Build history of the part. All positions in model axes, mm. Face numbers are marked on the shaded views. A direction names the side the tool comes from. Give positions to 0.01 mm unless a question says otherwise; leave off trailing zeros. Order: outer loops, then holes, each group sorted by start corner. A loop starts at its lowest first (then second) coordinate and runs counter-clockwise, first axis right, second up. Notation, with made-up numbers: M 0.5,22 L 59.5,22 A37 cw 59.5,60 Z; hole C -13.5,76 d6. An arc over 180 degrees is marked long. One line per item, written item: value.
from build123d import *

# Parameters (mm, degrees)
SKETCH1_W           = 96.52
SKETCH1_H           = 63.5
SKETCH1_R           = 1.905
BOSS_EXTRUDE1_DEPTH = 29.21
SKETCH2_W           = 86.36
SKETCH2_H           = 50.8
SKETCH2_W_2         = 5.705747077
SKETCH2_H_2         = 14.834942399
BOSS_EXTRUDE2_DEPTH = 2.54
SKETCH3_R           = 1.27
CUT_EXTRUDE1_DEPTH  = 2.54
SKETCH4_W           = 7.62
SKETCH4_H           = 6.35
SKETCH4_W_2         = 10.16
BOSS_EXTRUDE3_DEPTH = 10.16


with BuildPart() as part:
    # Sketch1 → Boss-Extrude1 (new body)
    with BuildSketch(Plane(origin=(0, 0, 0), x_dir=(1, 0, 0), z_dir=(0, 1, 0))):
        Rectangle(SKETCH1_W, SKETCH1_H)
        with Locations(Location((-43.18, 26.67, 0), (0, 0, 90))):
            Circle(SKETCH1_R, mode=Mode.SUBTRACT)
        with Locations(Location((43.18, 26.67, 0), (0, 0, 90))):
            Circle(SKETCH1_R, mode=Mode.SUBTRACT)
        with Locations(Location((43.18, -26.67, 0), (0, 0, 90))):
            Circle(SKETCH1_R, mode=Mode.SUBTRACT)
        with Locations(Location((-43.18, -26.67, 0), (0, 0, 90))):
            Circle(SKETCH1_R, mode=Mode.SUBTRACT)
    extrude(amount=BOSS_EXTRUDE1_DEPTH)

    # Sketch2 → Boss-Extrude2 (add)
    with BuildSketch(Plane(origin=(0, 29.21, 0), x_dir=(1, 0, 0), z_dir=(0, 1, 0))):
        with Locations((-3.048, -4.318)):
            Rectangle(SKETCH2_W, SKETCH2_H)
        with Locations((44.441430006, 9.82656441)):
            Rectangle(SKETCH2_W_2, SKETCH2_H_2)
    extrude(amount=BOSS_EXTRUDE2_DEPTH)

    # Sketch3 → Cut-Extrude1 (cut)
    with BuildSketch(Plane.XZ):
        with Locations(Location((-25.4, 12.7, 0), (0, 0, 270))):
            Circle(SKETCH3_R)
    extrude(amount=-CUT_EXTRUDE1_DEPTH, mode=Mode.SUBTRACT)

    # Sketch4 → Boss-Extrude3 (add)
    with BuildSketch(Plane(origin=(0, 0, -31.75), x_dir=(-1, 0, 0), z_dir=(0, 0, -1))):
        with Locations((-31.496, 10.287)):
            Rectangle(SKETCH4_W, SKETCH4_H)
        with Locations((-20.32, 10.287)):
            Rectangle(SKETCH4_W_2, SKETCH4_H)
        with Locations((-8.382, 10.287)):
            Rectangle(SKETCH4_W, SKETCH4_H)
        with Locations((2.54, 10.287)):
            Rectangle(SKETCH4_W_2, SKETCH4_H)
    extrude(amount=BOSS_EXTRUDE3_DEPTH)


solid = part.part
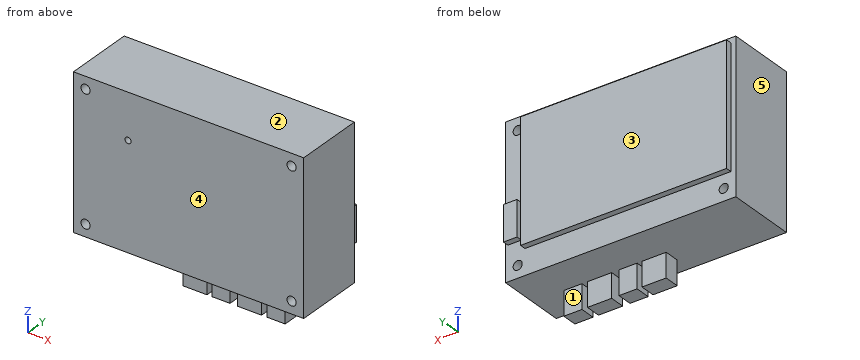
1) Saw through at A-A, the plane x = 43.18. Write the cut outline in (y, z) (3 decimals), then the cut area to 3 significant figures.
Check values:
outline: M 0,-31.75 L 29.21,-31.75 L 29.21,-28.575 L 0,-28.575 Z; M 0,-24.765 L 29.21,-24.765 L 29.21,-17.244 L 31.75,-17.244 L 31.75,-2.409 L 29.21,-2.409 L 29.21,24.765 L 0,24.765 Z; M 0,28.575 L 29.21,28.575 L 29.21,31.75 L 0,31.75 Z
area: 1,670 mm^2
2) Mould opens along Y. For the marked faces 3, 4 and 5 say: released by +Y, released by -Y, zero draft, split by the parting line, or undercut.
Check values:
face 3: released by +Y
face 4: released by -Y
face 5: zero draft
3) Pin check, flat tips, straight feed: pin 1 (2 mm diameter, centred on y = 31, z = 6, fed in from -X); pin 2 (2 mm diameter, centred on x = -7.5, y = 30.5, fed in from +Z); pin 3 (3 mm diameter, centred on x = -11.5, y = 30, fed in from -Z). Stop position of each tip, or through.
Check values:
pin 1: x = -46.23
pin 2: z = 29.72
pin 3: z = -31.75
4) Tool access for the marked faces 1 and 2: list every direction of +Z, -Z, +X, -X, +Y, -Y with a clear straight run to the whole face (end or side of a thin tool).
Check values:
face 1: -Z, +X, -X, +Y
face 2: +Z, +X, -X, +Y, -Y
5) Saw through at B-B, the plane z = -26.67. Write the cut outline in (x, y) (3 decimals), then the cut area to 3 significant figures.
Check values:
outline: M -48.26,0 L -45.085,0 L -45.085,29.21 L -48.26,29.21 Z; M -41.275,0 L 41.275,0 L 41.275,29.21 L -41.275,29.21 Z; M 45.085,0 L 48.26,0 L 48.26,29.21 L 45.085,29.21 Z
area: 2,600 mm^2
6) Drill centre lines: probe 1 along Z at (x, y) = (43.18, 21.75) (3 decimals); probe 2 along X at (y, z) = (9, -26.67) (3 decimals); probe 3 along Z at (x, y) = (-43.5, 18.5). Where is each one in solid material? Low to high. Write a range as from..to.
Check values:
probe 1: -31.75..-28.575, -24.765..24.765, 28.575..31.75
probe 2: -48.26..-45.085, -41.275..41.275, 45.085..48.26
probe 3: -31.75..-28.55, -24.79..24.79, 28.55..31.75
7) Saw through at D-D, the plane y = 19.5. Write the cut outline in (x, z) (3 decimals).
Check values:
outline: M -48.26,-31.75 L 48.26,-31.75 L 48.26,31.75 L -48.26,31.75 Z; hole C -43.18,-26.67 d3.81; hole C -43.18,26.67 d3.81; hole C 43.18,-26.67 d3.81; hole C 43.18,26.67 d3.81
8) Saw through at C-C, the plane z = 26.67. Write the cut outline in (x, y) (3 decimals), then the cut area to 3 significant figures.
Check values:
outline: M -48.26,0 L -45.085,0 L -45.085,29.21 L -41.275,29.21 L -41.275,0 L 41.275,0 L 41.275,29.21 L 40.132,29.21 L 40.132,31.75 L -46.228,31.75 L -46.228,29.21 L -48.26,29.21 Z; M 45.085,0 L 48.26,0 L 48.26,29.21 L 45.085,29.21 Z
area: 2,820 mm^2
